Could you check a few things on this drawing? It's one solid part, dimensions in mm from its lowest x, y, z. Give positions to 0.01 mm unless a question says otherwise; leave off trailing zeros. Order: outer loops, then holes, each group sorted by start corner. A loop starts at its lowest first (then second) coordinate and runs counter-clockwise, first axis right, second up. Notation, with made-up numbers: (76.5, -15.75) -> (102.5, -15.75) arc R33 cw to (102.5, 18.25) -> close; hole circle Ø8 at (26, 56). An arc over 180 degrees is marked (long way). Use one line per item in the form item = value. Start each with the question number.
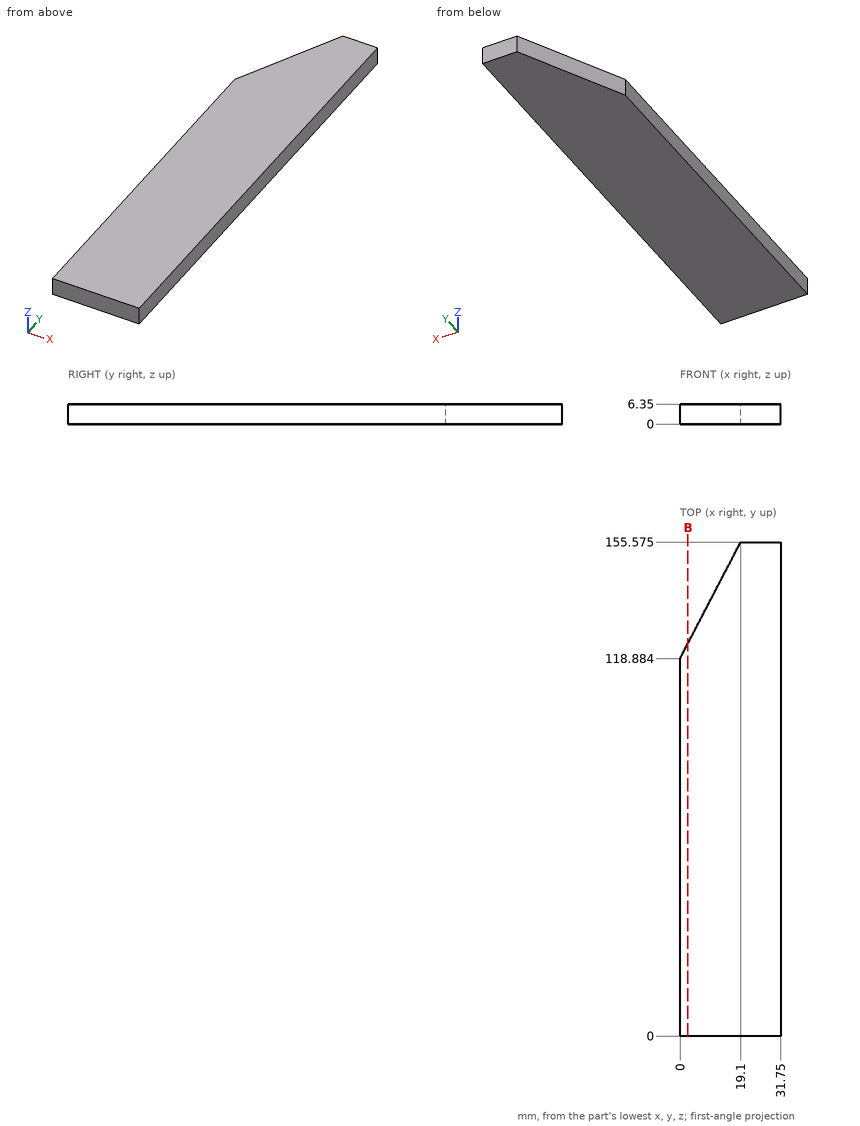
(1) Imagine slicing it at B-B (x = 2.5). Write out the boundary of the cut face in (y, z).
(2) I'm going to push a flat-ended pin straight in: pin 1 Ø1.5 at (x, z) = (22.5, 4) entering from -Y. Where does the tip first touch, or does it pass through?
(3) Please list where these lines run through material, in increasing order: probe 1 along Y at (x, z) = (17.5, 2) (1 decimal); probe 2 along X at (y, z) = (135, 3.75); probe 3 along Y at (x, z) = (12, 1.5) (1 decimal).
Calculated:
q1.outline = (0, 0) -> (123.69, 0) -> (123.69, 6.35) -> (0, 6.35) -> close
q2.pin_1 = 0
q3.probe_1 = 0 to 152.5
q3.probe_2 = 8.39 to 31.75
q3.probe_3 = 0 to 141.9
